```python
from build123d import *

# Parameters (mm, degrees)
F0_R      = 25
F1_DEPTH  = 270
F2_R      = 75
F3_DEPTH  = 50
F3_FACE_R = 75
F6_R      = 12.5
F9_R      = 12.5
F4_FACE_R = 75


with BuildPart() as f1:
    # F0 (on Front) → F1 (new body)
    with BuildSketch(Plane.XZ):
        Circle(F0_R)
    extrude(amount=F1_DEPTH)

    # F2 (on face) → F3 (join)
    with BuildSketch(Plane.XZ.offset(270)):
        Circle(F2_R)
    extrude(amount=F3_DEPTH)

    # F4: F1 across plane


with BuildPart() as f1_1:
    add(f1.part)
    add(f1.part.mirror(Plane.XZ))

    # F3_face (on face) → F7 section 0
    with BuildSketch(Plane.XZ.offset(320)):
        Circle(F3_FACE_R)
    # F6 (on offset) → F7 section 1
    with BuildSketch(Plane.XZ.offset(345)):
        Circle(F6_R)
    loft()

    # F9 (on offset) → F10 section 0
    with BuildSketch(Plane(origin=(0, 345, 0), x_dir=(-1, 0, 0), z_dir=(0, 1, 0))):
        Circle(F9_R)
    # F4_face (on face) → F10 section 1
    with BuildSketch(Plane(origin=(0, 320, 0), x_dir=(-1, 0, 0), z_dir=(0, 1, 0))):
        Circle(F4_FACE_R)
    loft()


solid = f1_1.part
```
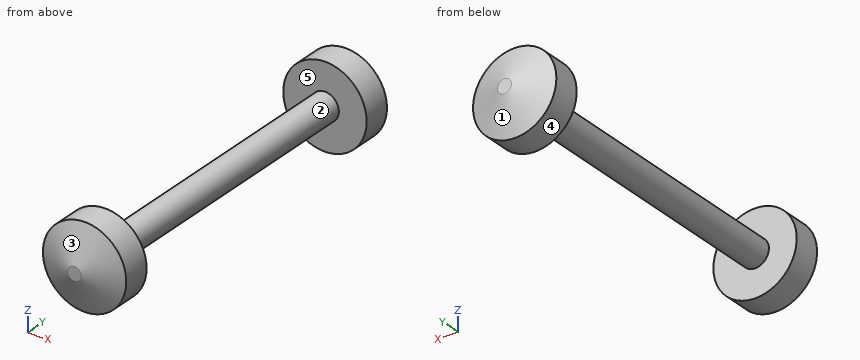
Source: CAD feature listing. Evaluate the final solid. Frame: model axes, mm. Face numbers are marked on the shaded views. A direction names the side the tool comes from. Round coordinates to 2 decimals unless told otherwise and drop trailing zeros. Loops run counter-clockwise (first coordinate to the right, second up) from the corner with the lowest first, then second, coordinate; pieces in that order, holes last. Notation, with made-up numbers: M 55,-13.75 L 102,-13.75 A14 ccw 102,7.25 Z; hole C -35,-26 d4. An arc over 180 degrees is marked long. Put each result on its own line as item: value.
(1) Access query for the marked faces 4 and 5. Directions: +Z, -Z, +X, -X, +Y, -Y. A direction counts if a zero-diameter tool reaches every point of the face in a straight line with its end or side. Return the directions, or none.
Solutions:
face 4: +Y, -Y
face 5: none
(2) First-contact query: pin 1 (2 mm diameter, centred on x = 47, z = -39, fed in from -Y); pin 2 (1.5 mm diameter, centred on x = -29, z = -6, fed in from -Y); pin 3 (8 mm diameter, centred on x = 35.5, z = 48, fed in from -Y). Flat tips, straight axial feed; report the tip coordinate or a pass-through.
Solutions:
pin 1: y = -325.97
pin 2: y = -338.45
pin 3: y = -327.72
(3) Ray query, line 1 (Y direction, x = -42, z = 40.5); line 2 (Y direction, x = 56, z = 26); line 3 (X direction, y = -295.5, z = 3). Return the intervals inside material, ascending. Write a range as [from, to].
Solutions:
line 1: [-326.66, -270], [270, 326.66]
line 2: [-325.3, -270], [270, 325.3]
line 3: [-74.94, 74.94]
(4) Section A-A, the plane x = 0. Return loops of the section in (y, z).
Solutions:
outline: M -345,-12.5 L -320,-75 L -270,-75 L -270,-25 L 270,-25 L 270,-75 L 320,-75 L 345,-12.5 L 345,12.5 L 320,75 L 270,75 L 270,25 L -270,25 L -270,75 L -320,75 L -345,12.5 Z
(5) Pull-direction query (Y, two-part tool) for the marked faces 1, 2 and 3; classes: released by +Y, released by -Y, zero draft, split by the parting line, or undercut.
Solutions:
face 1: released by +Y
face 2: undercut
face 3: released by -Y
(6) Section B-B, the plane y = -107.5. Return loops of the section in (x, z).
Solutions:
outline: C 0,0 d50
(7) Section C-C, the plane y = 286. Return loops of the section in (x, z).
Solutions:
outline: C 0,0 d150
